Model file for the job. Use its own axes, mm. A direction names the side the tool comes from. Round coordinates to 2 decimals unless told otherwise and drop trailing zeros. Order: outer loops, then holes, each group sorted by start corner. A loop starts at its lowest first (then second) coordinate and runs counter-clockwise, first axis right, second up. Notation, with made-up numbers: (66.25, 67.25) - (116.25, 67.25) arc R20 ccw to (116.25, 89.25) - close; hole circle Ø7 at (1, 59.5). An arc over 180 degrees is marked (long way). Put each result on its own line as item: value. Start each with the question number.
Item 1: Saw through at D-D on x = -10. List the corners of the cut face in (y, z), plus the area to 3 significant figures.
Item 2: Mould opens along Z. For faces 1 (the face through (-16, 4, 38.564)), 2 (the face through (15, 9, 38.564)), 3 (the face through (-11.142, 2.346, 43.529)), 4 (the face through (20, 13.5, 43)) say: pulls with the +Z half, pulls with the -Z half, needs draft (parallel to the pull), parting line crosses it, or undercut.
Item 3: Saw through at A-A on z = 43.25. List the corners of the cut face in (x, y), plus the area to 3 significant figures.
Item 4: Saw through at B-B on x = -2.5. List the corners of the cut face in (y, z), plus the area to 3 significant figures.
Item 5: Saw through at C-C on y = -6.75. List the corners of the cut face in (x, z), plus the area to 3 significant figures.
Item 6: Pin check, flat tips, straight feed: pin 1 Ø12 at (x, z) = (-15, 30.5) entering from -Y; pin 2 Ø1.2 at (x, y) = (-15.5, 4) entering from +Z; pin 3 Ø2.5 at (x, y) = (18, 9) entering from -Z. Stop position of each tip, or through.
Item 7: Probe probe 1 along X at (y, z) = (1.75, 44); probe 2 along Z at (x, y) = (10, -5.5); probe 3 along X at (y, z) = (6.5, 42.75). List the from-to ranges inside material, lowest first.
Item 8: Which spindle directions (+Z, -Z, +X, -X, +Y, -Y) get a long thin tool onto all of the face, cutting with end or side? Do faces 5 (the face through (7.136, 2.346, 43.398)), 6 (the face through (9, 5, 31)), 7 (the face through (-7.498, 1, 31)). Say none if no direction does.
Solid Edge part; units mm, degrees
sketch "Sketch1" plane through (0, 0, 0) normal (0, -1, 0) x (1, 0, 0)
  line L0 (-7.4976, 38.564) -> (42.5024, 38.564)
  line L1 (42.5024, 38.564) -> (42.5024, 23.564)
  line L2 (42.5024, 23.564) -> (-7.4976, 23.564)
  line L3 (-7.4976, 23.564) -> (-17.4976, 23.564)
  arc A0 (-17.4976, 38.564) -> (-17.4976, 23.564) centre (-17.4976, 31.064) ccw
  line L4 (-7.4976, 38.564) -> (-17.4976, 38.564)
  dimension "D1" = 7.4976
  dimension "D2" = 42.5024
extrude "Protrusion1" add sketch "Sketch1" against normal blind 5
sketch "Sketch2" plane through (17.5024, 2.5, 38.564) normal (0, 0, 1) x (1, 0, 0)
  line L0 (-31.5, 11) -> (25, 11)
  line L1 (25, 11) -> (25, -11)
  line L2 (25, -11) -> (-31.5, -11)
  line L3 (-31.5, -11) -> (-31.5, 11)
  dimension "D1" = 25
  dimension "D2" = 25
  dimension "D3" = 31.5
extrude "Extrusionsausprägung_4" add sketch "Sketch2" along normal blind 9
hole "Bohrung_1" at (2.5024, 0, 31.064) direction (0, 1, 0) diameter 4 end through all
hole "Hole1" at (28.5024, 0, 31.064) direction (0, 1, 0) diameter 4 end through all
sketch "Sketch3" plane through (8.7524, 0, 31.064) normal (0, -1, 0) x (1, 0, 0)
  line L0 (-26.25, 7.5) -> (-16.25, 7.5)
  line L1 (-16.25, 7.5) -> (-16.25, -7.5)
  line L2 (-16.25, -7.5) -> (-26.25, -7.5)
  arc A0 (-26.25, -7.5) -> (-26.25, 7.5) centre (-26.25, 0) cw
extrude "Extrusionsausschnitt_1" cut sketch "Sketch3" against normal blind 2.5
hole "Bohrung_4" at (-17.4976, 2.5, 31.064) direction (0, 1, 0) diameter 4 end through all
sketch "Sketch4" plane through (17.5024, -8.5, 43.064) normal (0, -1, 0) x (1, 0, 0)
  line L0 (-26, 4.5) -> (-13, 4.5)
  line L1 (-13, 4.5) -> (-13, 3.7601)
  arc A0 (-13, 3.7601) -> (-13.5, -2.5) centre (-13.5, 0.65) cw
  line L2 (-25.5, -2.5) -> (-13.5, -2.5)
  arc A1 (-26, 3.7601) -> (-25.5, -2.5) centre (-25.5, 0.65) ccw
  line L3 (-26, 4.5) -> (-26, 3.7601)
  dimension "D1" = 26
  dimension "D2" = 13
extrude "Cutout1" cut sketch "Sketch4" against normal through all
Results found:
1. outline: (-8.5, 38.56) - (2.5, 38.56) - (2.5, 23.56) - (5, 23.56) - (5, 38.56) - (13.5, 38.56) - (13.5, 41.28) - (-8.5, 41.28) - close; (-8.5, 46.15) - (13.5, 46.15) - (13.5, 47.56) - (-8.5, 47.56) - close
1. area: 129 mm²
2. face 1: pulls with the +Z half
2. face 2: pulls with the -Z half
2. face 3: undercut
2. face 4: needs draft
3. outline: (-14, -8.5) - (-11.11, -8.5) - (-11.11, 13.5) - (-14, 13.5) - close; (7.12, -8.5) - (42.5, -8.5) - (42.5, 13.5) - (7.12, 13.5) - close
3. area: 842 mm²
4. outline: (-8.5, 38.56) - (0, 38.56) - (0, 23.56) - (5, 23.56) - (5, 38.56) - (13.5, 38.56) - (13.5, 40.56) - (-8.5, 40.56) - close
4. area: 119 mm²
5. outline: (-14, 38.56) - (42.5, 38.56) - (42.5, 47.56) - (4.5, 47.56) - (4.5, 46.82) arc R3.15 cw to (4, 40.56) - (-8, 40.56) arc R3.15 cw to (-8.5, 46.82) - (-8.5, 47.56) - (-14, 47.56) - close
5. area: 393 mm²
6. pin 1: stops at y = 2.5
6. pin 2: stops at z = 38.56
6. pin 3: stops at z = 38.56
7. probe 1: x = -14 to -11.13, 7.14 to 42.5
7. probe 2: z = 38.56 to 47.56
7. probe 3: x = -14 to -11, 7 to 42.5
8. face 5: +Y, -Y
8. face 6: -Z, +X, -X, +Y
8. face 7: -Z, -X, -Y
